Could you check a few things on this drawing? It's one solid part, dimensions in mm from its lowest x, y, z. A direction names the side the tool comes from. Give positions to 0.01 mm unless a question says otherwise; leave off trailing zeros. Loops run counter-clockwise (first coordinate to the right, second up) from the corner with the lowest first, then second, coordinate; pieces in that order, holes last. Notation, with made-up numbers: (26, 18) - (67, 18) arc R18 cw to (67, 42) - close; hole circle Ø6 at (53.5, -7). An arc over 180 degrees is marked (long way). Write each question's results on one line, items separated by ' | '. Start each with the question number.
(1) Suppose I cut it at B-B (x = 13.5). Please give me the cut outline in (y, z), and give its area (3 significant figures).
(2) Suppose I cut it at D-D (x = 19). Please give me the cut outline in (y, z), and give its area (3 significant figures).
(3) I need wall thicknesses on line 1 (X direction, y = 18, z = 28); line 2 (X direction, y = 11.5, z = 4); line 3 (Y direction, x = 20, z = 13). Which ranges of each line are inside material? Lowest first, please.
(4) Suppose I cut it at C-C (z = 32). Please give me the cut outline in (x, y).
(5) Suppose I cut it at A-A (y = 17). Please give me the cut outline in (x, z), and give its area (3 significant figures).
(6) If we mould it in two halves opening along X, with no side actions, what happens to the marked faces 1, 2 and 3? For each: released by +X, released by -X, zero draft, split by the parting line, or undercut.
(7) On a 3-axis mill with a long thin cutter (end or side, diameter ignored), from which of +Z, -Z, +X, -X, +Y, -Y can I reach the whole of each face in a straight line? I mean the marked faces 4 and 5. Say none if no direction works.
(8) For pin 1 (12 mm diameter, centred on x = 5.5, z = 20.5, fed in from +Y); pin 2 (12 mm diameter, centred on x = 4, z = 24, fed in from +Y); pin 3 (8 mm diameter, centred on y = 26, z = 23, fed in from -X), each with a flat end and sliding along its axis, tell me the tip position at first contact or that it passes through.
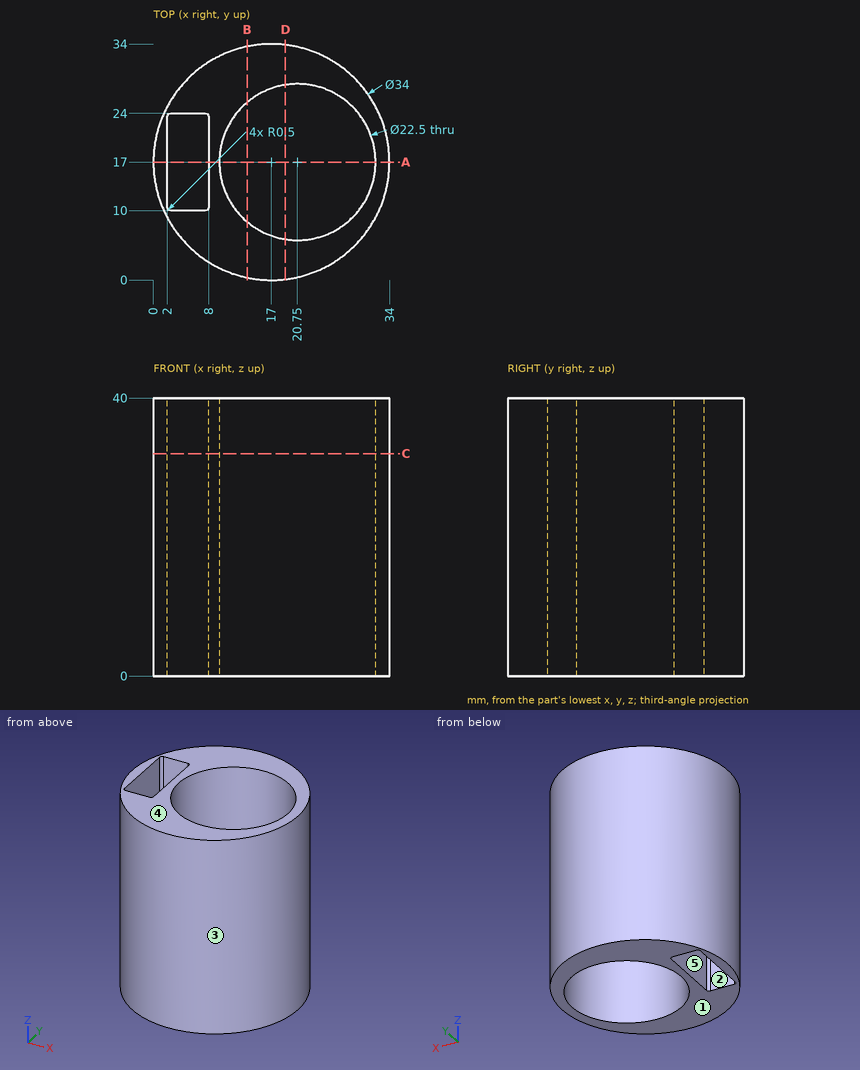
Output values:
1) outline: (0.36, 0) - (8.4, 0) - (8.4, 40) - (0.36, 40) - close; (25.6, 0) - (33.64, 0) - (33.64, 40) - (25.6, 40) - close | area: 643 mm2
2) outline: (0.12, 0) - (5.89, 0) - (5.89, 40) - (0.12, 40) - close; (28.11, 0) - (33.88, 0) - (33.88, 40) - (28.11, 40) - close | area: 462 mm2
3) line 1: 0.03 to 2, 8 to 9.54, 31.96 to 33.97 | line 2: 0.91 to 2, 8 to 10.94, 30.56 to 33.09 | line 3: 0.27 to 5.78, 28.22 to 33.73
4) outline: circle Ø34 at (17, 17); hole (2, 10.5) arc R0.5 ccw to (2.5, 10) - (7.5, 10) arc R0.5 ccw to (8, 10.5) - (8, 23.5) arc R0.5 ccw to (7.5, 24) - (2.5, 24) arc R0.5 ccw to (2, 23.5) - close; hole circle Ø22.5 at (20.75, 17)
5) outline: (0, 0) - (2, 0) - (2, 40) - (0, 40) - close; (8, 0) - (9.5, 0) - (9.5, 40) - (8, 40) - close; (32, 0) - (34, 0) - (34, 40) - (32, 40) - close | area: 220 mm2
6) face 1: zero draft | face 2: undercut | face 3: split by the parting line
7) face 4: +Z, +X, -X, +Y, -Y | face 5: +Z, -Z
8) pin 1: y = 33.09 | pin 2: y = 32.49 | pin 3: x = 0.75
